Here's the drawing with two shaded views (mm, measured from the low corner). I have some questions. Give positions to 0.01 mm unless a question says otherwise; leave off trailing zeros. Write each loop counter-clockwise with the first axis right and the second up, starting at its lowest first coordinate (ties: lowest second). Pieces come first, ordered by that corner, then holes. Notation, with made-up numbers: (25, 43.25) -> (54, 43.25) arc R27 cw to (54, 61.25) -> close; hole circle Ø9 at (-24.5, 39). An arc over 180 degrees is marked (long way). One line per item, written item: value.
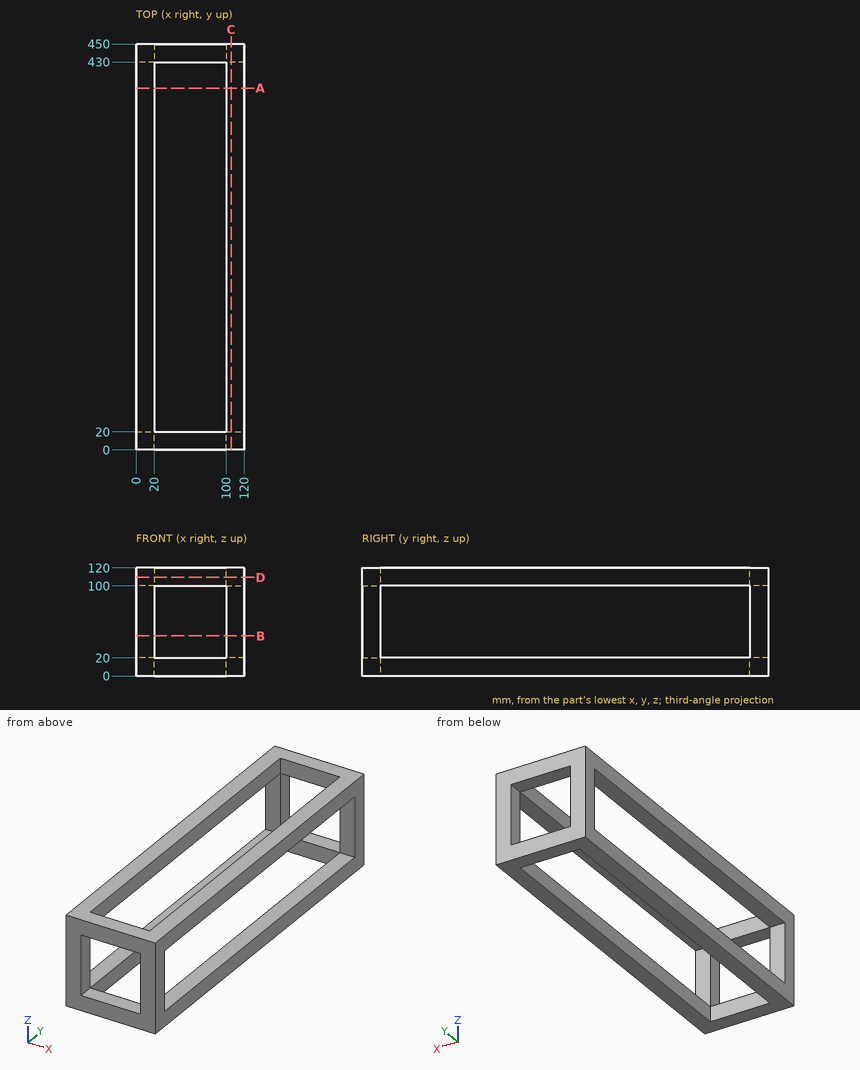
1) If we section it at A-A (y = 401): Write out the boundary of the cut face in (x, z), and give its area (3 significant figures).
Answer list:
outline: (0, 0) -> (20, 0) -> (20, 20) -> (0, 20) -> close; (0, 100) -> (20, 100) -> (20, 120) -> (0, 120) -> close; (100, 0) -> (120, 0) -> (120, 20) -> (100, 20) -> close; (100, 100) -> (120, 100) -> (120, 120) -> (100, 120) -> close
area: 1,600 mm^2
2) If we section it at C-C (x = 105.5): Write out the boundary of the cut face in (y, z).
Answer list:
outline: (0, 0) -> (450, 0) -> (450, 120) -> (0, 120) -> close; hole (20, 20) -> (430, 20) -> (430, 100) -> (20, 100) -> close
3) I need wall thicknesses on L1, parallel to Z at x = 111.5, y = 293; L2, parallel to Y at x = 25.5, z = 14.5. Which ranges of each line are inside material? Lowest first, please.
Answer list:
L1: z = 0 to 20, 100 to 120
L2: y = 0 to 20, 430 to 450
4) If we section it at B-B (z = 44.5): Write out the boundary of the cut face in (x, y), and give its area (3 significant figures).
Answer list:
outline: (0, 0) -> (20, 0) -> (20, 20) -> (0, 20) -> close; (0, 430) -> (20, 430) -> (20, 450) -> (0, 450) -> close; (100, 0) -> (120, 0) -> (120, 20) -> (100, 20) -> close; (100, 430) -> (120, 430) -> (120, 450) -> (100, 450) -> close
area: 1,600 mm^2
5) If we section it at D-D (z = 109.5): Write out the boundary of the cut face in (x, y), and give its area (3 significant figures).
Answer list:
outline: (0, 0) -> (120, 0) -> (120, 450) -> (0, 450) -> close; hole (20, 20) -> (100, 20) -> (100, 430) -> (20, 430) -> close
area: 21,200 mm^2
